Check sheet for the modelled part. Datum: model origin and axes. Units: mm. Round coordinates to 2 decimals unless told otherwise and drop trailing zeros. Loops run counter-clockwise (first coordinate to the right, second up) from the corner with the lowest first, then second, coordinate; pieces in that order, holes last. Notation, with made-up numbers: (81, -31) - (101, -31) arc R31 ccw to (101, -3) - close; hole circle Ø6 at (-29.75, 48). An arc over 180 degrees is marked (long way). Answer in a Markdown table with one row per item. Add a question column.
(1) Cross-section at B-B on z = 0. Enter the section's corners in (x, y).
(2) Cross-section at C-C on x = -127.5. Enter the section's corners in (y, z).
(3) Thickness scan on line 1 along X through (y, z) = (-1.05, 10); line 2 along Z through (x, y) = (-108, -0.85); line 3 along X through (y, z) = (-1.8, 28.5). Record the ranges inside material, lowest first.
(4) Cross-section at D-D on z = -31. Enter the section's corners in (x, y).
(5) Cross-section at A-A on y = -1.25. Enter the section's corners in (x, z), then the cut area to 3 significant figures.
from build123d import *

# Parameters (mm, degrees)
F1_DEPTH = 2
F2_R     = 2.25
F3_DEPTH = 2


with BuildPart() as f1:
    # F0 (on Front) → F1 (new body)
    with BuildSketch(Plane.XZ):
        with BuildLine():
            Line((-72.933308, -117.5), (147.066692, -117.5))
            Line((147.066692, -117.5), (147.066692, 117.5))
            Line((147.066692, 117.5), (-72.933308, 117.5))
            Line((-72.933308, 117.5), (-175.433308, 15))
            ThreePointArc((-175.433308, 15), (-160.433308, 0), (-175.433308, -15))
            Line((-175.433308, -15), (-72.933308, -117.5))
        make_face()
    extrude(amount=F1_DEPTH)

    # F2 (on face) → F3 (cut, through all)
    with BuildSketch(Plane.XZ.offset(2)):
        with BuildLine():
            Line((68.816692, -4.25), (80.316692, -4.25))
            ThreePointArc((80.316692, -4.25), (84.566692, 0), (80.316692, 4.25))
            Line((80.316692, 4.25), (68.816692, 4.25))
            ThreePointArc((68.816692, 4.25), (64.566692, 0), (68.816692, -4.25))
        make_face()
        with Locations((57.066692, -112.5)):
            Circle(F2_R)
        with Locations((57.066692, 112.5)):
            Circle(F2_R)
    extrude(amount=-F3_DEPTH, mode=Mode.SUBTRACT)


solid = f1.part
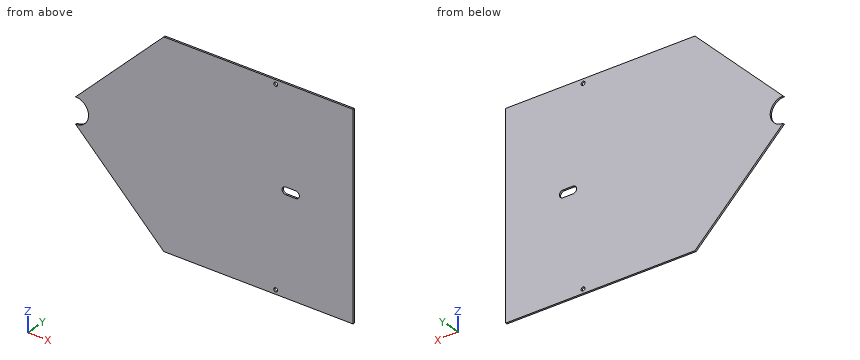
Answers:
| question | item | result |
|---|---|---|
| 1 | outline | (-160.43, -2) - (64.57, -2) - (64.57, 0) - (-160.43, 0) - close; (84.57, -2) - (147.07, -2) - (147.07, 0) - (84.57, 0) - close |
| 2 | outline | (-2, -62.93) - (0, -62.93) - (0, 62.93) - (-2, 62.93) - close |
| 3 | line 1 | x = -164.25 to 147.07 |
| 3 | line 2 | z = -82.43 to 82.43 |
| 3 | line 3 | x = -161.93 to 147.07 |
| 4 | outline | (-159.43, -2) - (147.07, -2) - (147.07, 0) - (-159.43, 0) - close |
| 5 | outline | (-175.43, -15) - (-72.93, -117.5) - (147.07, -117.5) - (147.07, 117.5) - (-72.93, 117.5) - (-175.43, 15) arc R15 cw to start; hole circle Ø4.5 at (57.07, -112.5); hole circle Ø4.5 at (57.07, 112.5); hole (68.82, -4.25) - (80.32, -4.25) arc R4.25 ccw to (80.32, 4.25) - (68.82, 4.25) arc R4.25 ccw to start |
| 5 | area | 64,700 mm^2 |
